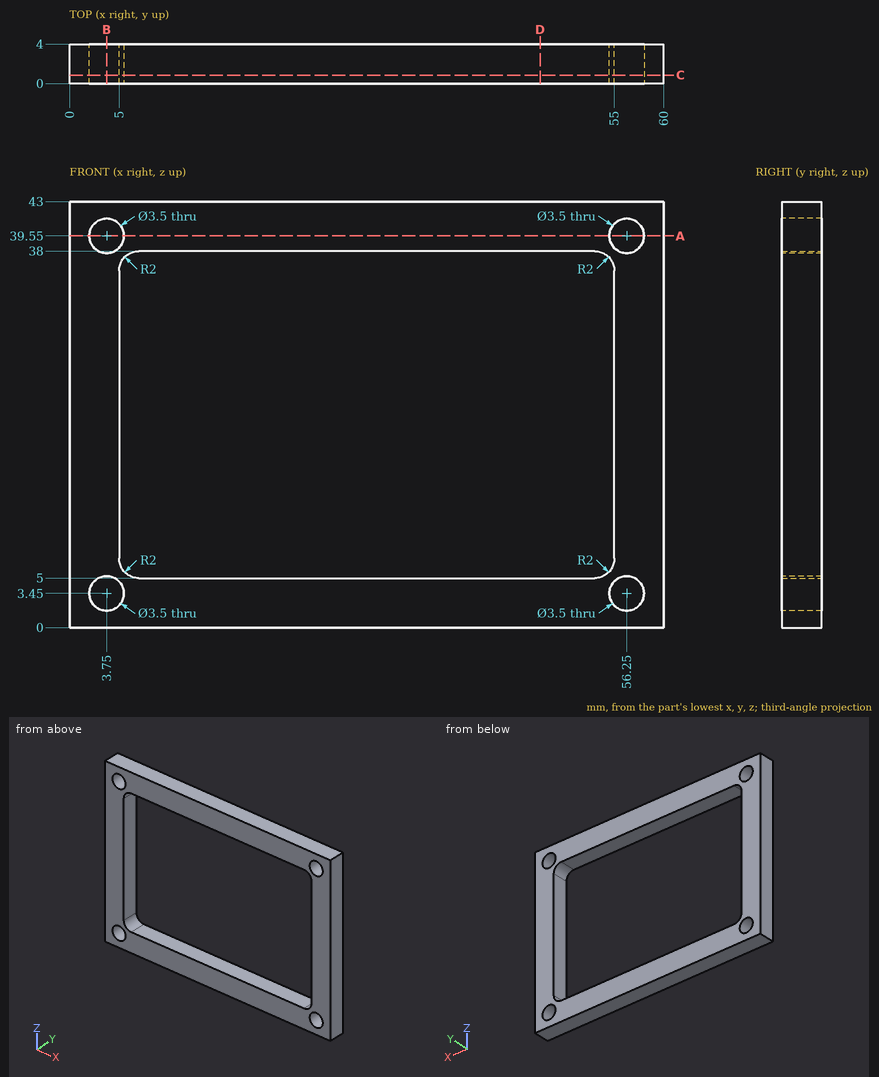
Geometry: see drawing. Coordinates: mm, zero at the bounding-box minimum. Give positions to 0.01 mm unless a question says otherwise; leave off trailing zeros. Loops run counter-clockwise (first coordinate to the right, second up) from the corner with the lowest first, then second, coordinate; pieces in that order, holes last. Notation, with made-up numbers: (26, -9) - (75, -9) arc R11 cw to (75, -2) - close; hole circle Ø4 at (41.25, -11). An arc over 180 degrees is marked (long way). Use CSV: the item, a comma, the result in double quotes. Start each with the question number.
1. Section D-D (x = 47.5). Output: boundary loops of the cut face in (y, z), then the cut area to 3 significant figures.
2. Ray query, L1, parallel to X at y = 2.4, z = 3.45; L2, parallel to Z at x = 3.75, y = 2.2; L3, parallel to X at y = 3.25, z = 17. Return the intervals inside material, ascending.
3. Section C-C (y = 0.85). Output: boundary loops of the cut face in (x, z).
4. Section A-A (z = 39.55). Output: boundary loops of the cut face in (x, y), then the cut area to 3 significant figures.
5. Section B-B (x = 3.75). Output: boundary loops of the cut face in (y, z).
Response:
1,outline,"(0, 0) - (4, 0) - (4, 5) - (0, 5) - close; (0, 38) - (4, 38) - (4, 43) - (0, 43) - close"
1,area,"40.0 mm²"
2,L1,"0 to 2, 5.5 to 54.5, 58 to 60"
2,L2,"0 to 1.7, 5.2 to 37.8, 41.3 to 43"
2,L3,"0 to 5, 55 to 60"
3,outline,"(0, 0) - (60, 0) - (60, 43) - (0, 43) - close; hole circle Ø3.5 at (3.75, 3.45); hole circle Ø3.5 at (3.75, 39.55); hole (5, 7) arc R2 ccw to (7, 5) - (53, 5) arc R2 ccw to (55, 7) - (55, 36) arc R2 ccw to (53, 38) - (7, 38) arc R2 ccw to (5, 36) - close; hole circle Ø3.5 at (56.25, 3.45); hole circle Ø3.5 at (56.25, 39.55)"
4,outline,"(0, 0) - (2, 0) - (2, 4) - (0, 4) - close; (5.5, 0) - (54.5, 0) - (54.5, 4) - (5.5, 4) - close; (58, 0) - (60, 0) - (60, 4) - (58, 4) - close"
4,area,"212 mm²"
5,outline,"(0, 0) - (4, 0) - (4, 1.7) - (0, 1.7) - close; (0, 5.2) - (4, 5.2) - (4, 37.8) - (0, 37.8) - close; (0, 41.3) - (4, 41.3) - (4, 43) - (0, 43) - close"
